CAD build for the part. Positions are in the model's coordinates, mm. A direction names the side the tool comes from. Coordinates: 2 decimals unless noted, no trailing zeros. Loops run counter-clockwise (first coordinate to the right, second up) from the corner with the lowest first, then second, coordinate; pieces in that order, holes last. Notation, with made-up numbers: (41.25, 54.5) -> (49.25, 54.5) arc R22 ccw to (49.25, 78.5) -> close; hole circle Ø10 at (41, 76.25). An arc over 180 degrees is marked (long way). Return JSON: item names as keys, results as strings. Group by question number.
(1) Probe L1, parallel to X at y = 5, z = 15; L2, parallel to Z at x = 15.5, y = 11.5; L3, parallel to Y at x = -29.5, z = -12. List the from-to ranges inside material, lowest first.
(2) Saw through at A-A on y = 6.25. Give the number of separate pieces and of enclosed holes in the cut face, then the cut area to 3 significant figures.
(3) Saw through at C-C on x = 0. Write the cut outline in (y, z).
(4) Mould opens along Z. For faces 4 (the face through (0, 28, 9)), 5 (the face through (-39.05, 0.99, -8.67)), 6 (the face through (-27.99, 3.84, -22.55)) say: pulls with the +Z half, pulls with the -Z half, needs draft (parallel to the pull), parting line crosses it, or undercut.
(5) Tool access for faces 1 (the face through (21, 14, 21)), 2 (the face through (-25.259, 9.916, -26.555)), 3 (the face through (-21, 17, -21)): list every direction of +Z, -Z, +X, -X, +Y, -Y with a clear straight run to the whole face (end or side of a thin tool).
(6) Saw through at B-B on z = 0. Write the cut outline in (x, y), then the cut area to 3 significant figures.
(7) Flat gauge pins, fed straight in: pin 1 Ø13 at (x, z) = (24, 19.5) entering from +Y; pin 2 Ø8 at (y, z) = (14, 17.5) entering from -X; pin 3 Ø2.5 at (x, z) = (21.5, -22.5) entering from -Y. Where does each tip first touch, or does it go through?
```python
from build123d import *

# Parameters (mm, degrees)
SKETCH1_R                 = 40
HOLDER_BASE_DEPTH         = 3
SKETCH2_R                 = 22
BALL_HOLDER_EXTRUDE_DEPTH = 25
SKETCH3_R                 = 7
PEG_EXTRUDES_DEPTH        = 14
SKETCH4_R                 = 5.25
PEG_HOLES_DEPTH           = 14
CHAMFER1_SIZE             = 1
CHAMFER2_SIZE             = 1


with BuildPart() as part:
    # Sketch1 → Holder Base (new body)
    with BuildSketch(Plane(origin=(0, 0, 0), x_dir=(1, 0, 0), z_dir=(0, 1, 0))):
        with Locations(Location((0, 0, 0), (0, 0, 270))):
            Circle(SKETCH1_R)
    extrude(amount=HOLDER_BASE_DEPTH)

    # Sketch2 → Ball Holder Extrude (add)
    with BuildSketch(Plane(origin=(0, 3, 0), x_dir=(1, 0, 0), z_dir=(0, 1, 0))):
        with Locations(Location((0, 0, 0), (0, 0, 270))):
            Circle(SKETCH2_R)
    extrude(amount=BALL_HOLDER_EXTRUDE_DEPTH)

    # Sketch5 → Ball Cut (revolve, cut)
    with BuildSketch(Plane.XY):
        with BuildLine():
            Line((0, 21.5865), (0, 34.4135))
            ThreePointArc((0, 34.4135), (-6.4135, 28), (0, 21.5865))
        make_face()
    revolve(axis=Axis((0, -1000, 0), (0, 1, 0)), mode=Mode.SUBTRACT)

    # Sketch3 → Peg Extrudes (add)
    with BuildSketch(Plane(origin=(0, 3, 0), x_dir=(1, 0, 0), z_dir=(0, 1, 0))):
        with Locations(Location((-21, 21, 0), (0, 0, 270))):
            Circle(SKETCH3_R)
        with Locations(Location((21, 21, 0), (0, 0, 270))):
            Circle(SKETCH3_R)
        with Locations(Location((21, -21, 0), (0, 0, 270))):
            Circle(SKETCH3_R)
        with Locations(Location((-21, -21, 0), (0, 0, 270))):
            Circle(SKETCH3_R)
    extrude(amount=PEG_EXTRUDES_DEPTH)

    # Sketch4 → Peg Holes (cut)
    with BuildSketch(Plane.XZ):
        with Locations(Location((-21, -21, 0), (0, 0, 270))):
            Circle(SKETCH4_R)
        with Locations(Location((-21, 21, 0), (0, 0, 270))):
            Circle(SKETCH4_R)
        with Locations(Location((21, 21, 0), (0, 0, 270))):
            Circle(SKETCH4_R)
        with Locations(Location((21, -21, 0), (0, 0, 270))):
            Circle(SKETCH4_R)
    extrude(amount=-PEG_HOLES_DEPTH, mode=Mode.SUBTRACT)

    # Chamfer1
    # the kernel refuses this chamfer: 1 mm, written as the material it adds along each edge
    with BuildSketch(Plane(origin=(-21, 3, -21), x_dir=(0, 0, 1), z_dir=(-1, 0, 0))) as chamfer1_piece_1:
        Polygon((7 + CHAMFER1_SIZE, 0), (7, CHAMFER1_SIZE), (7, 0), align=None)
    revolve(axis=Axis((-21, 3, -21), (0, 1, 0)))
    with BuildSketch(Plane(origin=(21, 3, -21), x_dir=(0, 0, 1), z_dir=(-1, 0, 0))) as chamfer1_piece_2:
        Polygon((7 + CHAMFER1_SIZE, 0), (7, CHAMFER1_SIZE), (7, 0), align=None)
    revolve(axis=Axis((21, 3, -21), (0, 1, 0)))
    with BuildSketch(Plane(origin=(21, 3, 21), x_dir=(0, 0, 1), z_dir=(-1, 0, 0))) as chamfer1_piece_3:
        Polygon((7 + CHAMFER1_SIZE, 0), (7, CHAMFER1_SIZE), (7, 0), align=None)
    revolve(axis=Axis((21, 3, 21), (0, 1, 0)))
    with BuildSketch(Plane(origin=(-21, 3, 21), x_dir=(0, 0, 1), z_dir=(-1, 0, 0))) as chamfer1_piece_4:
        Polygon((7 + CHAMFER1_SIZE, 0), (7, CHAMFER1_SIZE), (7, 0), align=None)
    revolve(axis=Axis((-21, 3, 21), (0, 1, 0)))
    with BuildSketch(Plane(origin=(0, 3, 0), x_dir=(0, 0, 1), z_dir=(-1, 0, 0))) as chamfer1_piece_5:
        Polygon((22 + CHAMFER1_SIZE, 0), (22, CHAMFER1_SIZE), (22, 0), align=None)
    revolve(axis=Axis((0, 3, 0), (0, 1, 0)))
    # the kernel refuses this chamfer: 1 mm, written as the material it takes off along each edge
    with BuildSketch(Plane(origin=(0, 28, 0), x_dir=(-1, 0, 0), z_dir=(0, 0, 1))) as chamfer1_2_piece_1:
        with BuildLine():
            Line((6.4135 + CHAMFER1_SIZE, 0), (6.319506315, 1.093993685))
            ThreePointArc((6.319506315, 1.093993685), (6.388622712, 0.564342173), (6.4135, 0))
            Line((6.4135, 0), (6.4135 + CHAMFER1_SIZE, 0))
        make_face()
    revolve(axis=Axis((0, 28, 0), (0, -1, 0)), mode=Mode.SUBTRACT)
    with BuildSketch(Plane(origin=(-21, 17, -21), x_dir=(0, 0, 1), z_dir=(-1, 0, 0))) as chamfer1_2_piece_2:
        Polygon((7, -CHAMFER1_SIZE), (7 - CHAMFER1_SIZE, 0), (7, 0), align=None)
    revolve(axis=Axis((-21, 17, -21), (0, 1, 0)), mode=Mode.SUBTRACT)
    with BuildSketch(Plane(origin=(21, 17, -21), x_dir=(0, 0, 1), z_dir=(-1, 0, 0))) as chamfer1_2_piece_3:
        Polygon((7, -CHAMFER1_SIZE), (7 - CHAMFER1_SIZE, 0), (7, 0), align=None)
    revolve(axis=Axis((21, 17, -21), (0, 1, 0)), mode=Mode.SUBTRACT)
    with BuildSketch(Plane(origin=(21, 17, 21), x_dir=(0, 0, 1), z_dir=(-1, 0, 0))) as chamfer1_2_piece_4:
        Polygon((7, -CHAMFER1_SIZE), (7 - CHAMFER1_SIZE, 0), (7, 0), align=None)
    revolve(axis=Axis((21, 17, 21), (0, 1, 0)), mode=Mode.SUBTRACT)
    with BuildSketch(Plane(origin=(-21, 17, 21), x_dir=(0, 0, 1), z_dir=(-1, 0, 0))) as chamfer1_2_piece_5:
        Polygon((7, -CHAMFER1_SIZE), (7 - CHAMFER1_SIZE, 0), (7, 0), align=None)
    revolve(axis=Axis((-21, 17, 21), (0, 1, 0)), mode=Mode.SUBTRACT)
    with BuildSketch(Plane(origin=(0, 3, 0), x_dir=(0, 0, 1), z_dir=(-1, 0, 0))) as chamfer1_2_piece_6:
        Polygon((40, -CHAMFER1_SIZE), (40 - CHAMFER1_SIZE, 0), (40, 0), align=None)
    revolve(axis=Axis((0, 3, 0), (0, 1, 0)), mode=Mode.SUBTRACT)
    with BuildSketch(Plane(origin=(0, 28, 0), x_dir=(0, 0, 1), z_dir=(-1, 0, 0))) as chamfer1_2_piece_7:
        Polygon((22, -CHAMFER1_SIZE), (22 - CHAMFER1_SIZE, 0), (22, 0), align=None)
    revolve(axis=Axis((0, 28, 0), (0, 1, 0)), mode=Mode.SUBTRACT)

    # Chamfer2
    chamfer2_edges = [part.edges().sort_by_distance(p)[0] for p in [
        (21, 14, -15.75),
        (21, 0, -15.75),
        (21, 14, 26.25),
        (21, 0, 26.25),
        (-21, 14, 26.25),
        (-21, 0, 26.25),
        (-21, 14, -15.75),
        (-21, 0, -15.75),
    ]]
    chamfer(chamfer2_edges, length=CHAMFER2_SIZE)


solid = part.part
```
Geometry results:
{
 "1": {"L1": "-24.61 to -17.39, -16.09 to 16.09, 17.39 to 24.61", "L2": "-25.33 to -16.67, -15.61 to 15.61, 16.67 to 25.33", "L3": "0 to 3"},
 "2": {"separate pieces": "5", "enclosed holes": "4", "area": "1,790 mm²"},
 "3": {"outline": "(0, -40) -> (2, -40) -> (3, -39) -> (3, -23) -> (4, -22) -> (27, -22) -> (28, -21) -> (28, -7.41) -> (26.91, -6.32) arc R6.41 cw to (26.91, 6.32) -> (28, 7.41) -> (28, 21) -> (27, 22) -> (4, 22) -> (3, 23) -> (3, 39) -> (2, 40) -> (0, 40) -> close"},
 "4": {"face 4": "needs draft", "face 5": "parting line crosses it", "face 6": "undercut"},
 "5": {"face 1": "-Y", "face 2": "+Y", "face 3": "-Z, -X, +Y"},
 "6": {"outline": "(-40, 0) -> (40, 0) -> (40, 2) -> (39, 3) -> (23, 3) -> (22, 4) -> (22, 27) -> (21, 28) -> (7.41, 28) -> (6.32, 26.91) arc R6.41 cw to (-6.32, 26.91) -> (-7.41, 28) -> (-21, 28) -> (-22, 27) -> (-22, 4) -> (-23, 3) -> (-39, 3) -> (-40, 2) -> close", "area": "1,270 mm²"},
 "7": {"pin 1": "y = 17", "pin 2": "x = -28", "pin 3": "y = 14"}
}
